Geometry check sheet. Reference: the model listing, model coordinates, mm. Face numbers are marked on the shaded views. A direction names the side the tool comes from. Round coordinates to 2 decimals unless told otherwise and drop trailing zeros. Loops run counter-clockwise (first coordinate to the right, second up) from the corner with the lowest first, then second, coordinate; pieces in that order, holes last. Notation, with made-up numbers: M -17,-4 L 13,-4 A18 ccw 13,5 Z; hole C -1.75,50 d2. An arc over 180 degrees is marked long. Write item = value, one per line.
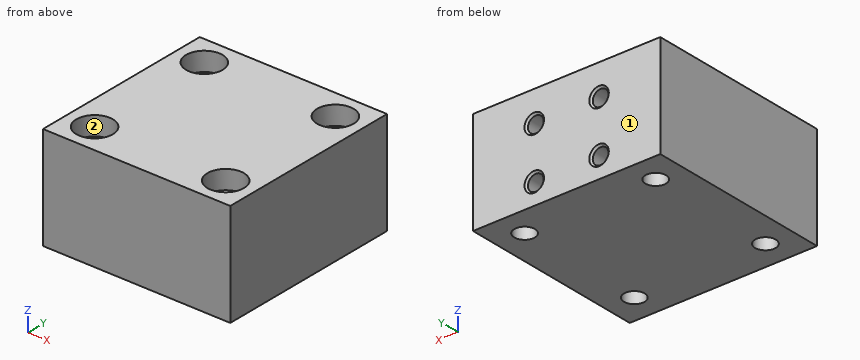
from build123d import *

# Parameters (mm, degrees)
F0_W           = 50
F0_H           = 50
F1_DEPTH       = 27.5
F3_D           = 5.5
F3_CBORE_D     = 9.75
F3_CBORE_DEPTH = 5
F5_D           = 4.2
F5_DEPTH       = 12
F5_CSINK_D     = 5.2
F5_CSINK_ANGLE = 90
F5_TIP         = 1.2618073


with BuildPart() as f1:
    # F0 (on Top) → F1 (new body)
    with BuildSketch(Plane.XY):
        Rectangle(F0_W, F0_H)
    extrude(amount=F1_DEPTH)

    # F3 (through all)
    with Locations(Plane.XY.offset(27.5)):
        with Locations((-17.5, 17.5), (17.5, 17.5), (-17.5, -17.5), (17.5, -17.5)):
            CounterBoreHole(F3_D / 2, F3_CBORE_D / 2, F3_CBORE_DEPTH)

    # F5
    with Locations(Plane(origin=(0, 25, 0), x_dir=(-1, 0, 0), z_dir=(0, 1, 0))):
        with Locations((-8.65, 19.35), (8.65, 19.35), (8.65, 5.65), (-8.65, 5.65)):
            CounterSinkHole(F5_D / 2, F5_CSINK_D / 2, depth=F5_DEPTH, counter_sink_angle=F5_CSINK_ANGLE)
            with Locations((0, 0, -(F5_DEPTH + F5_TIP / 2))):  # 118° drill point
                Cone(0, F5_D / 2, F5_TIP, mode=Mode.SUBTRACT)


solid = f1.part
(1) Sectioned sample at B-B on z = 2. Record the cut outline in (x, y), then the cut area to 3 significant figures.
Result set:
outline = M -25,-25 L 25,-25 L 25,25 L -25,25 Z; hole C -17.5,-17.5 d5.5; hole C -17.5,17.5 d5.5; hole C 17.5,-17.5 d5.5; hole C 17.5,17.5 d5.5
area = 2,400 mm2
(2) Sectioned sample at A-A on y = 17.5. Record the cut outline in (x, z) (3 decimals).
Result set:
outline = M -25,0 L -20.25,0 L -20.25,22.5 L -22.375,22.5 L -22.375,27.5 L -25,27.5 Z; M -14.75,0 L 14.75,0 L 14.75,22.5 L 12.625,22.5 L 12.625,27.5 L -12.625,27.5 L -12.625,22.5 L -14.75,22.5 Z; M 20.25,0 L 25,0 L 25,27.5 L 22.375,27.5 L 22.375,22.5 L 20.25,22.5 Z; hole C -8.65,5.65 d4.2; hole C -8.65,19.35 d4.2; hole C 8.65,5.65 d4.2; hole C 8.65,19.35 d4.2
(3) Sectioned sample at D-D on y = -17.5. Record the cut outline in (x, z) (3 decimals).
Result set:
outline = M -25,0 L -20.25,0 L -20.25,22.5 L -22.375,22.5 L -22.375,27.5 L -25,27.5 Z; M -14.75,0 L 14.75,0 L 14.75,22.5 L 12.625,22.5 L 12.625,27.5 L -12.625,27.5 L -12.625,22.5 L -14.75,22.5 Z; M 20.25,0 L 25,0 L 25,27.5 L 22.375,27.5 L 22.375,22.5 L 20.25,22.5 Z
(4) Tool access check on the marked faces 1 and 2. Record the directions out of +Z, -Z, +X, -X, +Y, -Y that give a thin tool (end or side, any length) a straight path to the whole face; none if there is none.
Result set:
face_1 = +Z, -Z, +X, -X, +Y
face_2 = +Z
(5) Depth check by flat-ended pin: pin 1 Ø3.5 at (x, y) = (17.5, 17.5) entering from +Z; pin 2 Ø8 at (x, y) = (-17.5, -17.5) entering from +Z. Enter the tip coordinate at first touch or a pass-through.
Result set:
pin_1 = through
pin_2 = 22.5
(6) Sectioned sample at C-C on x = 15.5. Record the cut outline in (y, z).
Result set:
outline = M -25,0 L -19.39,0 L -19.39,22.5 L -21.95,22.5 L -21.95,27.5 L -25,27.5 Z; M -15.61,0 L 15.61,0 L 15.61,22.5 L 13.05,22.5 L 13.05,27.5 L -13.05,27.5 L -13.05,22.5 L -15.61,22.5 Z; M 19.39,0 L 25,0 L 25,27.5 L 21.95,27.5 L 21.95,22.5 L 19.39,22.5 Z
(7) Material ranges on line 1 along Z through (x, y) = (8.65, 17.75); line 2 along X through (y, z) = (13, 19.25); line 3 along Y through (x, z) = (17.5, 24.15) (3 decimals), recorded low to high. Write a range as from..to.
Result set:
line_1 = 0..3.55, 7.75..17.25, 21.45..27.5
line_2 = -25..-10.75, -6.55..6.55, 10.75..25
line_3 = -25..-22.375, -12.625..12.625, 22.375..25
